from build123d import *

# Parameters (mm, degrees)
SKETCH1_W                     = 120
SKETCH1_H                     = 100
BOSS_EXTRUDE1_DEPTH           = 10
SKETCH2_W                     = 13
SKETCH2_H                     = 20
CUT_EXTRUDE1_DEPTH            = 37
SKETCH3_W                     = 14
SKETCH3_H                     = 10
SKETCH3_W_2                   = 7.5
CUT_EXTRUDE4_DEPTH            = 10
SKETCH10_R                    = 1.5
CUT_EXTRUDE5_DEPTH            = 75.5
CBORE_FOR_M3_SHCS_D           = 3.4
CBORE_FOR_M3_SHCS_DEPTH       = 23
CBORE_FOR_M3_SHCS_CBORE_D     = 6.5
CBORE_FOR_M3_SHCS_CBORE_DEPTH = 3
CBORE_FOR_M3_SHCS_TIP         = 1.021463052


with BuildPart() as part:
    # Sketch1 → Boss-Extrude1 (new body)
    with BuildSketch(Plane(origin=(0, 0, 0), x_dir=(1, 0, 0), z_dir=(0, 1, 0))):
        Rectangle(SKETCH1_W, SKETCH1_H)
    extrude(amount=BOSS_EXTRUDE1_DEPTH)

    # Sketch2 → Cut-Extrude1 (cut)
    with BuildSketch(Plane.XY.offset(50)):
        with Locations((-36, 0)):
            Rectangle(SKETCH2_W, SKETCH2_H)
        with Locations((-12, 0)):
            Rectangle(SKETCH2_W, SKETCH2_H)
        with Locations((12, 0)):
            Rectangle(SKETCH2_W, SKETCH2_H)
        with Locations((36, 0)):
            Rectangle(SKETCH2_W, SKETCH2_H)
    extrude(amount=-CUT_EXTRUDE1_DEPTH, mode=Mode.SUBTRACT)

    # Sketch3 → Cut-Extrude4 (cut)
    with BuildSketch(Plane.XY.offset(50)):
        with Locations((53, 5)):
            Rectangle(SKETCH3_W, SKETCH3_H)
        with Locations((25.75, 5)):
            Rectangle(SKETCH3_W_2, SKETCH3_H)
        with Locations((1.75, 5)):
            Rectangle(SKETCH3_W_2, SKETCH3_H)
        with Locations((-22.25, 5)):
            Rectangle(SKETCH3_W_2, SKETCH3_H)
    extrude(amount=-CUT_EXTRUDE4_DEPTH, mode=Mode.SUBTRACT)

    # Sketch10 → Cut-Extrude5 (cut)
    with BuildSketch(Plane(origin=(46, 0, 0), x_dir=(0, 0, -1), z_dir=(1, 0, 0))):
        with Locations((-45, 5)):
            Circle(SKETCH10_R)
    extrude(amount=-CUT_EXTRUDE5_DEPTH, mode=Mode.SUBTRACT)

    # CBORE for M3 SHCS
    with Locations(Plane(origin=(-676.293536786, 10, -1323.282701689), x_dir=(1, 0, 0), z_dir=(0, 1, 0))):
        with Locations((731.293536786, -1281.282701689), (731.293536786, -1343.282701689), (621.293536786, -1281.282701689), (621.293536786, -1365.282701689), (621.293536786, -1323.282701689), (731.293536786, -1312.282701689)):
            CounterBoreHole(CBORE_FOR_M3_SHCS_D / 2, CBORE_FOR_M3_SHCS_CBORE_D / 2, CBORE_FOR_M3_SHCS_CBORE_DEPTH, depth=CBORE_FOR_M3_SHCS_DEPTH)
            with Locations((0, 0, -(CBORE_FOR_M3_SHCS_DEPTH + CBORE_FOR_M3_SHCS_TIP / 2))):  # 118° drill point
                Cone(0, CBORE_FOR_M3_SHCS_D / 2, CBORE_FOR_M3_SHCS_TIP, mode=Mode.SUBTRACT)


solid = part.part
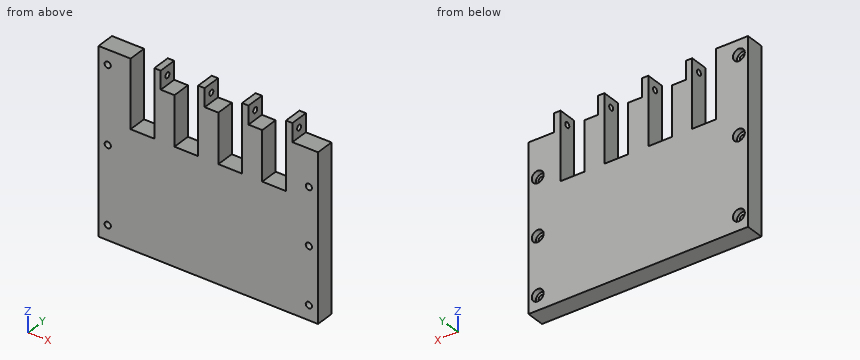
For this review, take the finished solid that the model builds, in its own axes (mm). Coordinates: 2 decimals unless noted, no trailing zeros. Order: outer loops, then holes, each group sorted by start corner. A loop starts at its lowest first (then second) coordinate and runs counter-clockwise, first axis right, second up. Notation, with made-up numbers: (-24.75, 80) - (29.25, 80) arc R30 cw to (29.25, 112) - close; hole circle Ø5 at (25.25, 70.5). An arc over 180 degrees is marked (long way). Answer as CSV lines item,"result". Start each with the question number.
1) Add section B-B (x = -55). State the section outline as (y, z) points, then the cut area to 3 significant figures.
2) Insertion check: P1, Ø2, axis at x = 39.5, y = 1, coming from the +Z side; P2, Ø4, axis at x = 26, y = 7, coming from the +Z side; P3, Ø4.5, axis at x = 55, z = -11, coming from the +Y side; P4, Ø8.5, axis at x = -55, z = 42, coming from the -Y side. Each pin has a flat end and moves straight along its axis. Give the tip position at first contact, or say it passes through.
3) Add section C-C (z = 0). State the section outline as (x, y) points.
4) To check wall thickness, follow line 1 along X through (y, z) = (3, -42); line 2 along X through (y, z) = (7.65, -42); line 3 along Z through (x, y) = (-55, 3). State the ranges of each line that lie inside material, in increasing order. Write a range as [from, to].
5) Add section A-A (z = -42). State the section outline as (x, y) points.
6) Add section D-D (y = 8.5). Count the separate pieces of the cut face and the enclosed holes in it, then the cut area to 3 significant figures.
Result:
1,outline,"(0, -50) - (10, -50) - (10, -45.25) - (7, -45.25) - (7, -43.7) - (0, -43.7) - close; (0, -40.3) - (7, -40.3) - (7, -38.75) - (10, -38.75) - (10, -3.25) - (7, -3.25) - (7, -1.7) - (0, -1.7) - close; (0, 1.7) - (7, 1.7) - (7, 3.25) - (10, 3.25) - (10, 38.75) - (7, 38.75) - (7, 40.3) - (0, 40.3) - close; (0, 43.7) - (7, 43.7) - (7, 45.25) - (10, 45.25) - (10, 50) - (0, 50) - close"
1,area,"870 mm^2"
2,P1,"z = 13"
2,P2,"z = 40"
2,P3,"y = 7"
2,P4,"y = 0"
3,outline,"(-60, 0) - (-56.7, 0) - (-56.7, 7) - (-58.25, 7) - (-58.25, 10) - (-60, 10) - close; (-53.3, 0) - (60, 0) - (60, 10) - (-51.75, 10) - (-51.75, 7) - (-53.3, 7) - close"
4,line 1,"[-60, -56.7], [-53.3, 53.3], [56.7, 60]"
4,line 2,"[-60, -58.25], [-51.75, 51.75], [58.25, 60]"
4,line 3,"[-50, -43.7], [-40.3, -1.7], [1.7, 40.3], [43.7, 50]"
5,outline,"(-60, 0) - (-56.7, 0) - (-56.7, 7) - (-58.25, 7) - (-58.25, 10) - (-60, 10) - close; (-53.3, 0) - (53.3, 0) - (53.3, 7) - (51.75, 7) - (51.75, 10) - (-51.75, 10) - (-51.75, 7) - (-53.3, 7) - close; (56.7, 0) - (60, 0) - (60, 10) - (58.25, 10) - (58.25, 7) - (56.7, 7) - close"
6,separate pieces,"1"
6,enclosed holes,"6"
6,area,"9,510 mm^2"
